from build123d import *

# Parameters (mm, degrees)
F0_W      = 38
F0_H      = 29
F1_DEPTH  = 2
F2_W      = 2
F2_H      = 36
F3_DEPTH  = 7.3
F4_R      = 2
F5_R      = 0.5
F6_R      = 2.5
F7_R      = 5
F7_R_2    = 1.25
F8_DEPTH  = 25
F9_R      = 1.25
F10_DEPTH = 25
F11_R     = 1.025
F12_DEPTH = 25
F13_R     = 1.25
F14_DEPTH = 25
F15_R     = 1.025
F16_DEPTH = 25
F17_R     = 1.3
F18_DEPTH = 51.6


with BuildPart() as f1:
    # F0 (on Right) → F1 (new body)
    with BuildSketch(Plane.YZ):
        Rectangle(F0_W, F0_H)
    extrude(amount=F1_DEPTH)

    # F2 (on face) → F3 (join)
    with BuildSketch(Plane.YZ.offset(2)):
        with Locations((18, -3.5)):
            Rectangle(F2_W, F2_H)
        with Locations((-18, -3.5)):
            Rectangle(F2_W, F2_H)
    extrude(amount=F3_DEPTH)

    # F4
    f4_edges = [f1.edges().sort_by_distance(p)[0] for p in [
        (9.3, -18, -21.5),
        (9.3, 18, -21.5),
        (9.3, 18, 14.5),
        (9.3, -18, 14.5),
    ]]
    fillet(f4_edges, radius=F4_R)

    # F5
    f5_edges = [f1.edges().sort_by_distance(p)[0] for p in [
        (2, -17, 0),
        (2, 17, 0),
    ]]
    fillet(f5_edges, radius=F5_R)

    # F6
    f6_edges = [f1.edges().sort_by_distance(p)[0] for p in [
        (0, -19, 0),
        (0, 19, 0),
    ]]
    fillet(f6_edges, radius=F6_R)

    # F7 (on face) → F8 (cut)
    with BuildSketch(Plane.YZ.offset(2)):
        Circle(F7_R)
        with Locations((0, -11)):
            Circle(F7_R_2)
        with Locations((7.7781745931, -7.7781745931)):
            Circle(F7_R_2)
        with Locations((11, 0)):
            Circle(F7_R_2)
        with Locations((7.7781745931, 7.7781745931)):
            Circle(F7_R_2)
        with Locations((0, 11)):
            Circle(F7_R_2)
        with Locations((-7.7781745931, 7.7781745931)):
            Circle(F7_R_2)
        with Locations((-11, 0)):
            Circle(F7_R_2)
        with Locations((-7.7781745931, -7.7781745931)):
            Circle(F7_R_2)
    extrude(amount=-F8_DEPTH, mode=Mode.SUBTRACT)

    # F9 (on face) → F10 (cut)
    with BuildSketch(Plane.YZ.offset(2)):
        with Locations((-11.4357154532, -5.1210655213)):
            Circle(F9_R)
        with Locations((5.1210655213, -11.4357154532)):
            Circle(F9_R)
        with Locations((11.4357154532, 5.1210655213)):
            Circle(F9_R)
        with Locations((-5.1210655213, 11.4357154532)):
            Circle(F9_R)
    extrude(amount=-F10_DEPTH, mode=Mode.SUBTRACT)

    # F11 (on face) → F12 (cut)
    with BuildSketch(Plane.YZ.offset(2)):
        with Locations((-7.9929938994, 3.5156610366)):
            Circle(F11_R)
        with Locations((-3.5156610366, -7.9929938994)):
            Circle(F11_R)
        with Locations((7.9929938994, -3.5156610366)):
            Circle(F11_R)
        with Locations((3.5156610366, 7.9929938994)):
            Circle(F11_R)
    extrude(amount=-F12_DEPTH, mode=Mode.SUBTRACT)

    # F13 (on face) → F14 (cut)
    with BuildSketch(Plane.YZ.offset(2)):
        with Locations((-7.9459964827, -3.6206303175)):
            Circle(F13_R)
        with Locations((3.6206303175, -7.9459964827)):
            Circle(F13_R)
        with Locations((7.9459964827, 3.6206303175)):
            Circle(F13_R)
        with Locations((-3.6206303175, 7.9459964827)):
            Circle(F13_R)
    extrude(amount=-F14_DEPTH, mode=Mode.SUBTRACT)

    # F15 (on face) → F16 (cut)
    with BuildSketch(Plane.YZ.offset(2)):
        with Locations((-10.8599086511, 6.4697190889)):
            Circle(F15_R)
        with Locations((-6.4697190889, -10.8599086511)):
            Circle(F15_R)
        with Locations((10.8599086511, -6.4697190889)):
            Circle(F15_R)
        with Locations((6.4697190889, 10.8599086511)):
            Circle(F15_R)
    extrude(amount=-F16_DEPTH, mode=Mode.SUBTRACT)

    # F17 (on face) → F18 (cut)
    with BuildSketch(Plane.XZ.offset(19)):
        with Locations((6.7, 10.469)):
            Circle(F17_R)
        with Locations((6.7, 3.924)):
            Circle(F17_R)
        with Locations((6.7, -12.546)):
            Circle(F17_R)
        with Locations((6.7, -19.091)):
            Circle(F17_R)
    extrude(amount=-F18_DEPTH, mode=Mode.SUBTRACT)


solid = f1.part
CAD build for the part. Positions are in the model's coordinates, mm. A direction names the side the tool comes from. Give positions to 0.01 mm unless a question says otherwise; leave off trailing zeros. Order: outer loops, then holes, each group sorted by start corner. A loop starts at its lowest first (then second) coordinate and runs counter-clockwise, first axis right, second up. Notation, with made-up numbers: (6.25, 54.5) -> (30.25, 54.5) arc R13 cw to (30.25, 62.5) -> close; hole circle Ø7 at (-1.75, -22). An arc over 180 degrees is marked (long way). Return JSON: item names as keys, results as strings.
Q1. Saw through at B-B (z = 0). Write the cut outline in (x, y), then the cut area to 3 significant figures.
Working result:
{"outline": "(0, -16.5) arc R2.5 ccw to (2.5, -19) -> (9.3, -19) -> (9.3, -17) -> (2.5, -17) arc R0.5 cw to (2, -16.5) -> (2, -12.25) -> (0, -12.25) -> close; (0, -9.75) -> (2, -9.75) -> (2, -5) -> (0, -5) -> close; (0, 5) -> (2, 5) -> (2, 9.75) -> (0, 9.75) -> close; (0, 12.25) -> (2, 12.25) -> (2, 16.5) arc R0.5 cw to (2.5, 17) -> (9.3, 17) -> (9.3, 19) -> (2.5, 19) arc R2.5 ccw to (0, 16.5) -> close", "area": "72.6 mm²"}
Q2. Saw through at C-C (y = 0). Write the cut outline in (x, z), then the cut area to 3 significant figures.
Working result:
{"outline": "(0, -14.5) -> (2, -14.5) -> (2, -12.25) -> (0, -12.25) -> close; (0, -9.75) -> (2, -9.75) -> (2, -5) -> (0, -5) -> close; (0, 5) -> (2, 5) -> (2, 9.75) -> (0, 9.75) -> close; (0, 12.25) -> (2, 12.25) -> (2, 14.5) -> (0, 14.5) -> close", "area": "28.0 mm²"}
Q3. Drill centre lines: line 1 (Z direction, x = 1.5, y = 0); line 2 (Y direction, x = 3, z = -1); line 3 (Z direction, x = 1.35, y = -11). Where is each one in solid material? Low to high.
Working result:
{"line 1": "-14.5 to -12.25, -9.75 to -5, 5 to 9.75, 12.25 to 14.5", "line 2": "-19 to -17, 17 to 19", "line 3": "-14.5 to -6.29, -3.95 to -1.25, 1.25 to 5.45, 7.49 to 14.5"}
Q4. Saw through at A-A (x = 3). Write the cut outline in (y, z).
Working result:
{"outline": "(-19, -21.5) -> (-17, -21.5) -> (-17, 14.5) -> (-19, 14.5) -> close; (17, -21.5) -> (19, -21.5) -> (19, 14.5) -> (17, 14.5) -> close"}
Q5. Which spindle directions (+Z, -Z, +X, -X, +Y, -Y) get a long thin tool onto all of the face, cutting with end or side? Do faces 1 (the face through (1.01, -12.36, -4.28)), 2 (the face through (2, -18, -18)). Say none if no direction does.
Working result:
{"face 1": "+X, -X", "face 2": "-Z, -X, +Y, -Y"}
Q6. Flat gauge pins, fed straight in: pin 1 (1.5 mm diameter, centred on x = 1.5, z = -8, fed in from -Y); pin 2 (1.6 mm diameter, centred on y = -18.5, z = -19.5, fed in from -X); pin 3 (13 mm diameter, centred on y = 0, z = 0, fed in from +X). Where does each tip first touch, or does it go through?
Working result:
{"pin 1": "y = -18.99", "pin 2": "x = 2", "pin 3": "x = 2"}
Q7. Saw through at D-D (y = -8). Write the cut outline in (x, z).
Working result:
{"outline": "(0, -14.5) -> (2, -14.5) -> (2, -9.01) -> (0, -9.01) -> close; (0, -6.55) -> (2, -6.55) -> (2, -4.87) -> (0, -4.87) -> close; (0, -2.37) -> (2, -2.37) -> (2, 2.49) -> (0, 2.49) -> close; (0, 4.54) -> (2, 4.54) -> (2, 6.55) -> (0, 6.55) -> close; (0, 9.01) -> (2, 9.01) -> (2, 14.5) -> (0, 14.5) -> close"}
Q8. Mould opens along Y. For faces 3 (the face through (6, 19, -4)), 4 (the face through (1, 6.8, 7)), 5 (the face through (7.9, 17.99, 9.97)) say: pulls with the +Y half, pulls with the -Y half, needs draft (parallel to the pull), parting line crosses it, or undercut.
Working result:
{"face 3": "pulls with the +Y half", "face 4": "undercut", "face 5": "needs draft"}
